Could you check a few things on this model? Use its own coordinates, in mm. A direction names the side the tool comes from. Give positions to 0.01 mm unless a question says otherwise; leave off trailing zeros. Loops run counter-clockwise (first coordinate to the right, second up) from the corner with the lowest first, then second, coordinate; pieces in that order, holes last. Notation, with made-up numbers: (42.25, -11) - (50.25, -11) arc R38 ccw to (50.25, 27) - close; hole circle Ø1 at (-2.75, -25). An arc over 180 degrees is marked (long way). Write each question's results on one line, items separated by ' | '. Start each with the question number.
1) I want a section at C-C, the plane y = 53.5. Write out the boundary of the cut face in (x, z), and give its area (3 significant figures).
2) If I drill on probe 1 along X at (y, z) = (-23.25, 0); probe 2 along Y at (x, z) = (-42, 1.5); probe 3 along Z at (x, y) = (-38, -25), over which ranges is the centre line in solid material (lowest first)? Write a range as [from, to].
3) On a 3-axis mill with a long thin cutter (end or side, diameter ignored), from which of +Z, -Z, +X, -X, +Y, -Y can I reach the whole of each face in a straight line? I mean faces 4 (the face through (-38, 72.797, 0)), 5 (the face through (-41.445, -21.408, -0.439)), 6 (the face through (-17.74, -10.99, 2.97)). Say none if no direction works.
4) If we mould it in two halves opening along Z, with no side actions, what happens to faces 1 (the face through (-12.52, 50.49, 0.11)), 2 (the face through (-26, 23, 7.5)), 3 (the face through (-38, -8.103, 0))? For each: +Z half, -Z half, draft (parallel to the pull), parting line (faces both ways), or undercut.
5) I want a section at A-A, the plane x = -38.1. Write out the boundary of the cut face in (y, z), and give its area (3 significant figures).
6) I'm going to push flat-ended pins straight in: pin 1 (8 mm diameter, centred on x = -12.7, z = 0, fed in from +Y); pin 2 (3.5 mm diameter, centred on x = -11.5, z = 0.5, fed in from +Y); pin 3 (8 mm diameter, centred on y = 62, z = -5, fed in from +X). Where does each tip first touch, or does it pass through?
from build123d import *

# Parameters (mm, degrees)
BOSS_EXTRUDE1_DEPTH                       = 7.5
CUT_EXTRUDE1_START                        = -10
CUT_EXTRUDE1_DEPTH                        = 5.7
SKETCH5_W                                 = 3.373501
SKETCH5_H                                 = 31.997045256
CUT_EXTRUDE2_START                        = -15
CUT_EXTRUDE2_DEPTH                        = 5.7
SKETCH8_W                                 = 3.373501
SKETCH8_H                                 = 15
F_17_64_0_26563_DIAMETER_HOLE2_AT_2_COUNT = 2
F_17_64_0_26563_DIAMETER_HOLE2_AT_2_PITCH = 25.4
CUT_EXTRUDE3_DEPTH                        = 10.2


with BuildPart() as part:
    # Sketch1 → Boss-Extrude1 (new, symmetric)
    with BuildSketch(Plane.XY):
        Polygon((0, -28.802954744), (0, 28.802954744), (-25.4, 72.797045256), (-50.8, 72.797045256), (-50.8, -28.802954744), (-25.4, -28.802954744), align=None)
    extrude(amount=BOSS_EXTRUDE1_DEPTH, both=True)

    # Sketch2 → Cut-Extrude1 (cut)
    with BuildSketch(Plane(origin=(12.472045256, 7.200738686, 0), x_dir=(0, 0, -1), z_dir=(0.8660254037844379, 0.5000000000000013, 0)).offset(CUT_EXTRUDE1_START)):
        Polygon((0, 34.055117767), (5.1, 36.999604139), (5.1, 42.888576885), (5.1, 45.833063258), (0, 45.833063258), (-5.1, 45.833063258), (-5.1, 42.888576885), (-5.1, 36.999604139), align=None)
    extrude(amount=-CUT_EXTRUDE1_DEPTH, mode=Mode.SUBTRACT)

    # Sketch5 → 17/64 (0.26563) Diameter Hole1 (revolve, cut)
    with BuildSketch(Plane(origin=(-16.160254038, 36.793335801, 0), x_dir=(0.500000000000001, -0.866025403784438, 0), z_dir=(0, 0, 1))):
        with Locations((1.6867505, 15.998522628)):
            Rectangle(SKETCH5_W, SKETCH5_H)
    revolve(axis=Axis((-21.659515352, 33.618335801, 0), (0.866025403784438, 0.5000000000000009, 0)), mode=Mode.SUBTRACT)

    # Sketch6 → Cut-Extrude2 (cut)
    with BuildSketch(Plane.XZ.offset(28.802954744).offset(CUT_EXTRUDE2_START)):
        Polygon((-31.34500185, 0), (-34.722500925, 5.85), (-41.477499075, 5.85), (-44.85499815, 0), (-41.477499075, -5.85), (-34.722500925, -5.85), align=None)
        Polygon((-9.322500925, 5.85), (-16.077499075, 5.85), (-19.45499815, 0), (-16.077499075, -5.85), (-9.322500925, -5.85), (-5.94500185, 0), align=None)
    extrude(amount=-CUT_EXTRUDE2_DEPTH, mode=Mode.SUBTRACT)

    # Sketch8 → 17/64 (0.26563) Diameter Hole2 (revolve, cut)
    with BuildSketch(Plane(origin=(-12.7, -13.802954744, 0), x_dir=(0, 0, 1), z_dir=(1, 0, 0))):
        with Locations((1.6867505, 7.5)):
            Rectangle(SKETCH8_W, SKETCH8_H)
    f_17_64_0_26563_diameter_hole2 = revolve(axis=Axis((-12.7, -7.452954744, 0), (0, -1, 0)), mode=Mode.SUBTRACT)

    # 17/64 (0.26563) Diameter Hole2 at 2: 17/64 (0.26563) Diameter Hole2 ×2
    with Locations(*[(-i * F_17_64_0_26563_DIAMETER_HOLE2_AT_2_PITCH, 0, 0) for i in range(1, F_17_64_0_26563_DIAMETER_HOLE2_AT_2_COUNT)]):
        add(f_17_64_0_26563_diameter_hole2, mode=Mode.SUBTRACT)

    # Sketch9 → Cut-Extrude3 (cut)
    with BuildSketch(Plane(origin=(0, 0, 5.1), x_dir=(-1, 0, 0), z_dir=(0, 0, -1))):
        Polygon((19.104740411, 41.893335801), (24.041085212, 41.893335801), (24.041085212, 39.043335801), align=None)
    extrude(amount=CUT_EXTRUDE3_DEPTH, mode=Mode.SUBTRACT)


solid = part.part
Answers:
1) outline: (-50.8, -7.5) - (-14.26, -7.5) - (-14.26, 7.5) - (-50.8, 7.5) - close | area: 548 mm2
2) probe 1: x = [-50.8, -41.47], [-34.73, -16.07], [-9.33, 0] | probe 2: y = [-28.8, -13.8], [-8.1, 72.8] | probe 3: z = [-7.5, -3.37], [3.37, 7.5]
3) face 4: +Z, -Z, +X, -X, +Y | face 5: -Y | face 6: none
4) face 1: draft | face 2: +Z half | face 3: undercut
5) outline: (-28.8, -7.5) - (72.8, -7.5) - (72.8, 7.5) - (-28.8, 7.5) - (-28.8, 3.37) - (-13.8, 3.37) - (-13.8, 5.85) - (-8.1, 5.85) - (-8.1, -5.85) - (-13.8, -5.85) - (-13.8, -3.37) - (-28.8, -3.37) - close | area: 1,360 mm2
6) pin 1: stops at y = 57.73 | pin 2: stops at y = 51.75 | pin 3: stops at x = -16.86
